Build history of the part. All positions in model axes, mm. Give positions to 0.01 mm unless a question says otherwise; leave off trailing zeros. Loops run counter-clockwise (first coordinate to the right, second up) from the corner with the lowest first, then second, coordinate; pieces in that order, holes last. Notation, with made-up numbers: (44, -30.75) -> (79, -30.75) arc R29 cw to (79, -7.75) -> close; hole circle Ø8 at (45, -39.5). An arc over 180 degrees is marked (long way). One line per question, with ' | ' between items. Start each with the question number.
(1) Flat gauge pins, fed straight in: pin 1 Ø2 at (y, z) = (-4.5, -8.5) entering from +X; pin 2 Ø10 at (x, z) = (-19.5, -13.5) entering from +Y. Where does each tip first touch, or does it go through?
(2) Slice it at B-B, the plane z = -5. Write the cut outline in (x, y), then the cut area to 3 significant figures.
(3) Slice it at A-A, the plane y = -4.75. Write the cut outline in (x, z), then the cut area to 3 significant figures.
(4) Slice it at C-C, the plane z = 2.5. Write the cut outline in (x, y).
(5) Drill centre lines: L1, parallel to X at y = -0.5, z = 8.5; L2, parallel to X at y = -5, z = -6; L3, parallel to Z at x = 62.5, y = -4.5. Where is each one in solid material? Low to high. Write a range as from..to.
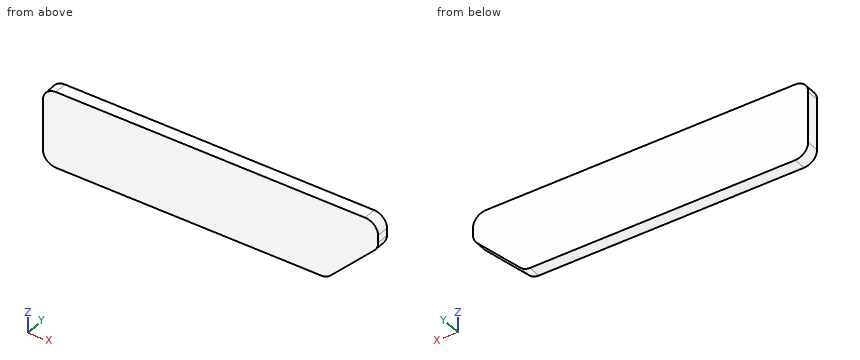
```python
from build123d import *

# Parameters (mm, degrees)
F1_DEPTH = 6.35


with BuildPart() as f1:
    # F0 (on Front) → F1 (new body)
    with BuildSketch(Plane.XZ):
        with BuildLine():
            ThreePointArc((82.55, 12.7), (80.690128, 17.190128), (76.2, 19.05))
            Line((76.2, 19.05), (-76.2, 19.05))
            ThreePointArc((-76.2, 19.05), (-80.690128, 17.190128), (-82.55, 12.7))
            Line((-82.55, 12.7), (-82.55, -12.7))
            ThreePointArc((-82.55, -12.7), (-80.690128, -17.190128), (-76.2, -19.05))
            Line((-76.2, -19.05), (54.519744, -19.05))
            ThreePointArc((54.519744, -19.05), (56.949784, -18.566635), (59.009872, -17.190128))
            Line((59.009872, -17.190128), (80.690128, 4.490128))
            ThreePointArc((80.690128, 4.490128), (82.066635, 6.550216), (82.55, 8.980256))
            Line((82.55, 8.980256), (82.55, 12.7))
        make_face()
    extrude(amount=F1_DEPTH)


solid = f1.part
```
Final values:
1) pin 1: x = 68.7 | pin 2: y = 0
2) outline: (-82.55, -6.35) -> (71.2, -6.35) -> (71.2, 0) -> (-82.55, 0) -> close | area: 976 mm2
3) outline: (-82.55, -12.7) arc R6.35 ccw to (-76.2, -19.05) -> (54.52, -19.05) arc R6.35 ccw to (59.01, -17.19) -> (80.69, 4.49) arc R6.35 ccw to (82.55, 8.98) -> (82.55, 12.7) arc R6.35 ccw to (76.2, 19.05) -> (-76.2, 19.05) arc R6.35 ccw to (-82.55, 12.7) -> close | area: 5,940 mm2
4) outline: (-82.55, -6.35) -> (78.7, -6.35) -> (78.7, 0) -> (-82.55, 0) -> close
5) L1: -82.55..82.53 | L2: -82.55..70.2 | L3: -13.7..19.05
